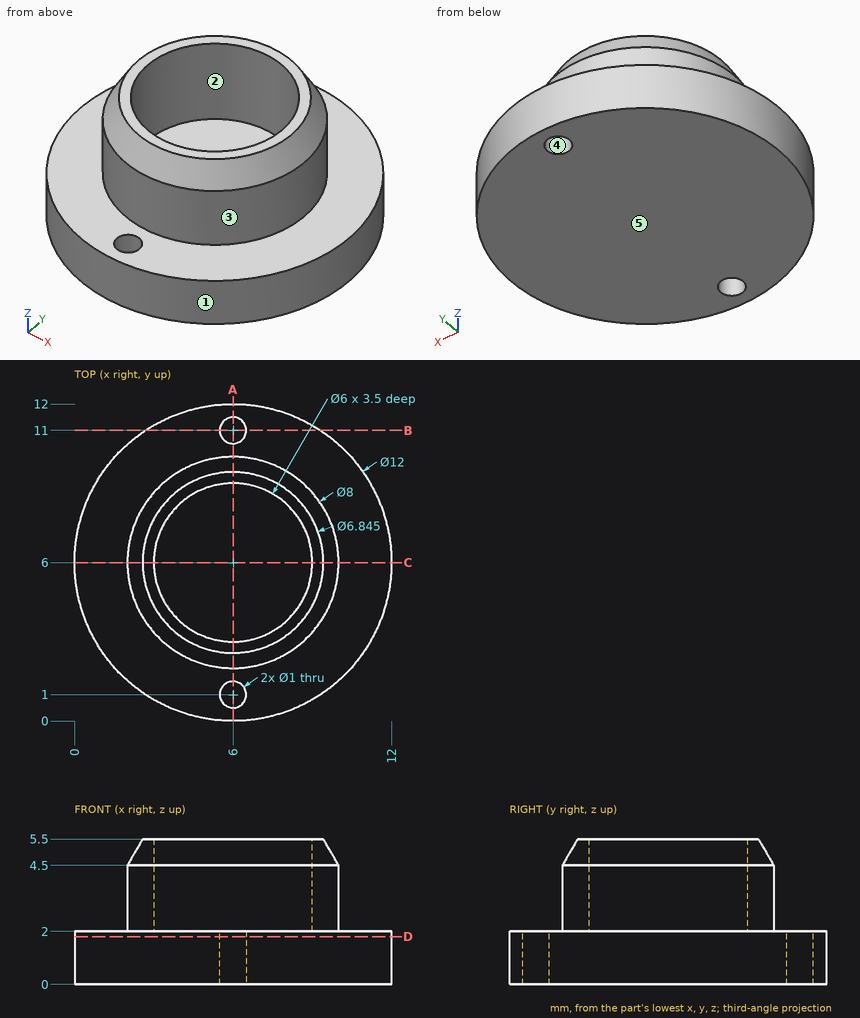
Here's the drawing with two shaded views (mm, measured from the low corner). I have some questions. A direction names the side the tool comes from. Coordinates: 2 decimals unless noted, no trailing zeros. Order: outer loops, then holes, each group sorted by start corner. A loop starts at its lowest first (then second) coordinate and runs counter-clockwise, first axis right, second up.
Q1. Suppose I cut it at C-C on y = 6. Please give me the cut outline in (x, z).
Q2. Will these pins go through, and if not, where does the flat tip stop? pin 1 (5 mm diameter, centred on x = 10.5, y = 2.5, fed in from -Z); pin 2 (1.5 mm diameter, centred on y = 4.5, z = 4, fed in from -X).
Q3. Suppose I cut it at D-D on z = 1.8. Please give me the cut outline in (x, y).
Q4. Please list where these lines run through material, in increasing order: L1, parallel to Y at x = 6, z = 1.5; L2, parallel to Y at x = 6, z = 4.15; L3, parallel to Z at x = 5, y = 1.75.
Q5. Which directions (+Z, -Z, +X, -X, +Y, -Y) give clear straight access to the entire face, cutting with the end or side of a thin tool? Please do the marked faces 1 and 2.
Q6. Suppose I cut it at B-B on y = 11. Please give me the cut outline in (x, z), and give its area (3 significant figures).
Q7. Thinking about a two-plate mould opening in Y: for the marked faces 3, 4 and 5, which applies, released by +Y, released by -Y, zero draft, split by the parting line, or undercut?
Q8. Suppose I cut it at A-A on x = 6. Please give me the cut outline in (y, z).
Answer:
1. outline: (0, 0) - (12, 0) - (12, 2) - (10, 2) - (10, 4.5) - (9.42, 5.5) - (9, 5.5) - (9, 2) - (3, 2) - (3, 5.5) - (2.58, 5.5) - (2, 4.5) - (2, 2) - (0, 2) - close
2. pin 1: stops at z = 0
2. pin 2: stops at x = 2.07
3. outline: circle Ø12 at (6, 6); hole circle Ø1 at (6, 1); hole circle Ø1 at (6, 11)
4. L1: y = 0 to 0.5, 1.5 to 10.5, 11.5 to 12
4. L2: y = 2 to 3, 9 to 10
4. L3: z = 0 to 2
5. face 1: +Z, -Z
5. face 2: +Z
6. outline: (2.68, 0) - (5.5, 0) - (5.5, 2) - (2.68, 2) - close; (6.5, 0) - (9.32, 0) - (9.32, 2) - (6.5, 2) - close
6. area: 11.3 mm2
7. face 3: split by the parting line
7. face 4: undercut
7. face 5: zero draft
8. outline: (0, 0) - (0.5, 0) - (0.5, 2) - (0, 2) - close; (1.5, 0) - (10.5, 0) - (10.5, 2) - (10, 2) - (10, 4.5) - (9.42, 5.5) - (9, 5.5) - (9, 2) - (3, 2) - (3, 5.5) - (2.58, 5.5) - (2, 4.5) - (2, 2) - (1.5, 2) - close; (11.5, 0) - (12, 0) - (12, 2) - (11.5, 2) - close
